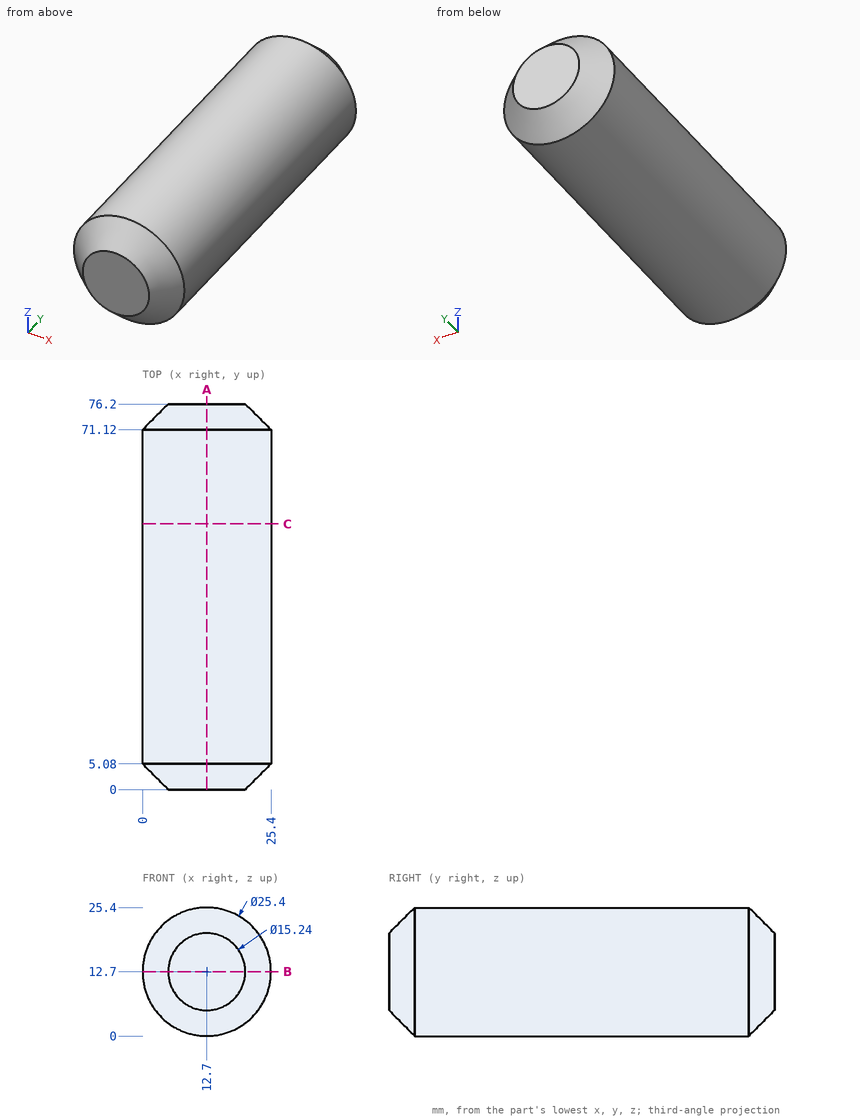
Input: dimensioned drawing with shaded views. Units: mm. Origin: part minimum x, y, z. Coordinates: 2 decimals unless noted, no trailing zeros. Loops run counter-clockwise (first coordinate to the right, second up) from the corner with the lowest first, then second, coordinate; pieces in that order, holes last. Notation, with made-up numbers: (29.25, 22.25) -> (38.25, 22.25) arc R20 ccw to (38.25, 61.25) -> close; hole circle Ø6 at (-9.5, 9). An arc over 180 degrees is marked (long way). Use a Markdown table: item, result. Add a question column.
(1) Section query B-B, the plane z = 12.7. Return loops of the section in (x, y), plus the area to 3 significant figures.
(2) Pin query (flat end, axial travel): pin 1 Ø2 at (x, y) = (22, 22.5) entering from +Z; pin 2 Ø1.5 at (y, z) = (55, 10.5) entering from +X; pin 3 Ø3 at (x, z) = (21, 15) entering from +Y; pin 4 Ø3 at (x, y) = (5.5, 56.5) entering from -Z. Return the tip coordinate at first contact, or that it passes through.
(3) Line query: line 1 along Z through (x, y) = (12.25, 11.5); line 2 along X through (y, z) = (67.5, 12.5); line 3 along X through (y, z) = (10.5, 18). Output: solid intervals per line, ascending.
(4) Section query A-A, the plane x = 12.7. Return loops of the section in (y, z), plus the area to 3 significant figures.
(5) Section query C-C, the plane y = 52.5. Return loops of the section in (x, z), plus the area to 3 significant figures.
Answer:
| question | item | result |
|---|---|---|
| 1 | outline | (0, 5.08) -> (5.08, 0) -> (20.32, 0) -> (25.4, 5.08) -> (25.4, 71.12) -> (20.32, 76.2) -> (5.08, 76.2) -> (0, 71.12) -> close |
| 1 | area | 1,880 mm^2 |
| 2 | pin 1 | stops at z = 22.31 |
| 2 | pin 2 | stops at x = 25.32 |
| 2 | pin 3 | stops at y = 76.2 |
| 2 | pin 4 | stops at z = 1.35 |
| 3 | line 1 | z = 0.01 to 25.39 |
| 3 | line 2 | x = 0 to 25.4 |
| 3 | line 3 | x = 1.16 to 24.24 |
| 4 | outline | (0, 5.08) -> (5.08, 0) -> (71.12, 0) -> (76.2, 5.08) -> (76.2, 20.32) -> (71.12, 25.4) -> (5.08, 25.4) -> (0, 20.32) -> close |
| 4 | area | 1,880 mm^2 |
| 5 | outline | circle Ø25.4 at (12.7, 12.7) |
| 5 | area | 507 mm^2 |
